Input: part model. Units: mm. Frame: model coordinates. A direction names the side the tool comes from. Coordinates: 2 decimals unless noted, no trailing zeros. Order: outer loops, then holes, each group sorted by start corner. A loop starts at its lowest first (then second) coordinate and runs counter-clockwise, first axis right, second up. Notation, with made-up numbers: (35, -24) -> (42, -24) arc R19 cw to (42, -13) -> close; hole circle Ø3 at (-3.5, -10). An arc over 180 degrees is marked (long way). Write each question's results on one line, items separated by ' | '.
```python
from build123d import *

# Parameters (mm, degrees)
BOSS_EXTRUDE1_DEPTH   = 35
F_2_0MM_DOWEL_HOLE1_D = 2


with BuildPart() as part:
    # Sketch2 → Boss-Extrude1 (new body)
    with BuildSketch(Plane.XY):
        Polygon((0, 0), (48.5, 0), (48.5, 3.5), (3.5, 3.5), (3.5, 39.5), (48.5, 39.5), (48.5, 43), (0, 43), align=None)
    extrude(amount=BOSS_EXTRUDE1_DEPTH)

    # Ø2.0mm Dowel Hole1 (through all)
    with Locations(Plane.XY.offset(35)):
        with Locations((46.557508768, 1.980929828), (1.882524811, 1.980929828), (1.882524811, 41.139003015), (46.557508768, 41.139003015)):
            Hole(F_2_0MM_DOWEL_HOLE1_D / 2)


solid = part.part
```
(1) Pin query (flat end, axial travel): P1, Ø10.5, axis at y = 18, z = 18.5, coming from the +X side. Return the tip coordinate at first contact, or that it passes through.
Return value:
P1: x = 3.5
(2) Cut plane B-B, the plane z = 2.5. Return loops of the section in (x, y), plus the area to 3 significant figures.
Return value:
outline: (0, 0) -> (48.5, 0) -> (48.5, 3.5) -> (3.5, 3.5) -> (3.5, 39.5) -> (48.5, 39.5) -> (48.5, 43) -> (0, 43) -> close; hole circle Ø2 at (1.88, 1.98); hole circle Ø2 at (1.88, 41.14); hole circle Ø2 at (46.56, 1.98); hole circle Ø2 at (46.56, 41.14) | area: 453 mm2
(3) Cut plane A-A, the plane x = 26.5. Return loops of the section in (y, z), plus the area to 3 significant figures.
Return value:
outline: (0, 0) -> (3.5, 0) -> (3.5, 35) -> (0, 35) -> close; (39.5, 0) -> (43, 0) -> (43, 35) -> (39.5, 35) -> close | area: 245 mm2
(4) Mould query, pull axis X, two halves, no side actions, for faces 1 (the face through (45.604, 2.281, 17.255)), 2 (the face through (26, 3.5, 17)), 3 (the face through (0, 22, 17)), 4 (the face through (48.5, 41, 17)). Classes: +X half, -X half, draft (parallel to the pull), parting line (faces both ways), or undercut.
Return value:
face 1: undercut | face 2: draft | face 3: -X half | face 4: +X half
(5) Cut plane C-C, the plane y = 5. Return loops of the section in (x, z), plus the area to 4 significant figures.
Return value:
outline: (0, 0) -> (3.5, 0) -> (3.5, 35) -> (0, 35) -> close | area: 122.5 mm2
(6) Line query: line 1 along Y through (x, z) = (39.5, 33); line 2 along X through (y, z) = (22, 23.5). Output: solid intervals per line, ascending. Write a range as from..to.
Return value:
line 1: 0..3.5, 39.5..43 | line 2: 0..3.5
(7) Reachability of faces 5 (the face through (26, 39.5, 17)), 6 (the face through (2.099, 1.005, 17.255)) from +Z, -Z, +X, -X, +Y, -Y: full face, straight path, thin tool, end or side. Return the list, or none.
Return value:
face 5: +Z, -Z, +X | face 6: +Z, -Z
